Source: three-view drawing plus pictorial views. Frame: mm from the lowest corner of the part. A direction names the side the tool comes from. Give positions to 0.01 mm unless a question says otherwise; leave off trailing zeros. Order: outer loops, then holes, each group sorted by start corner. A loop starts at its lowest first (then second) coordinate and runs counter-clockwise, first axis right, second up. Notation, with made-up numbers: M -22.75,8 L 1.25,8 A29 ccw 1.25,37 Z; hole C 58,-39 d9. An arc over 180 degrees is marked long. Use CSV: the item, a comma, the result in double quotes. Start each with the question number.
Item 1: Section query A-A on y = 23. Return loops of the section in (x, z).
Item 2: Access query for the marked faces 1 and 2. Directions: +Z, -Z, +X, -X, +Y, -Y. A direction counts if a zero-diameter tool reaches every point of the face in a straight line with its end or side. Return the directions, or none.
Item 3: Section query B-B on z = 3.1. Return loops of the section in (x, y).
Item 4: Ray query, probe 1 along Y at (x, z) = (10, 2.35); probe 2 along Y at (x, z) = (14.75, 2.2); probe 3 along Y at (x, z) = (13, 4). Return the intervals inside material, ascending. Write a range as from..to.
Item 5: Section query C-C on x = 13.15. Return loops of the section in (y, z).
Item 6: Pull-direction query (X, two-part tool) for the marked faces 3, 4 and 5; classes: +X half, -X half, draft (parallel to the pull), parting line (faces both ways), or undercut.
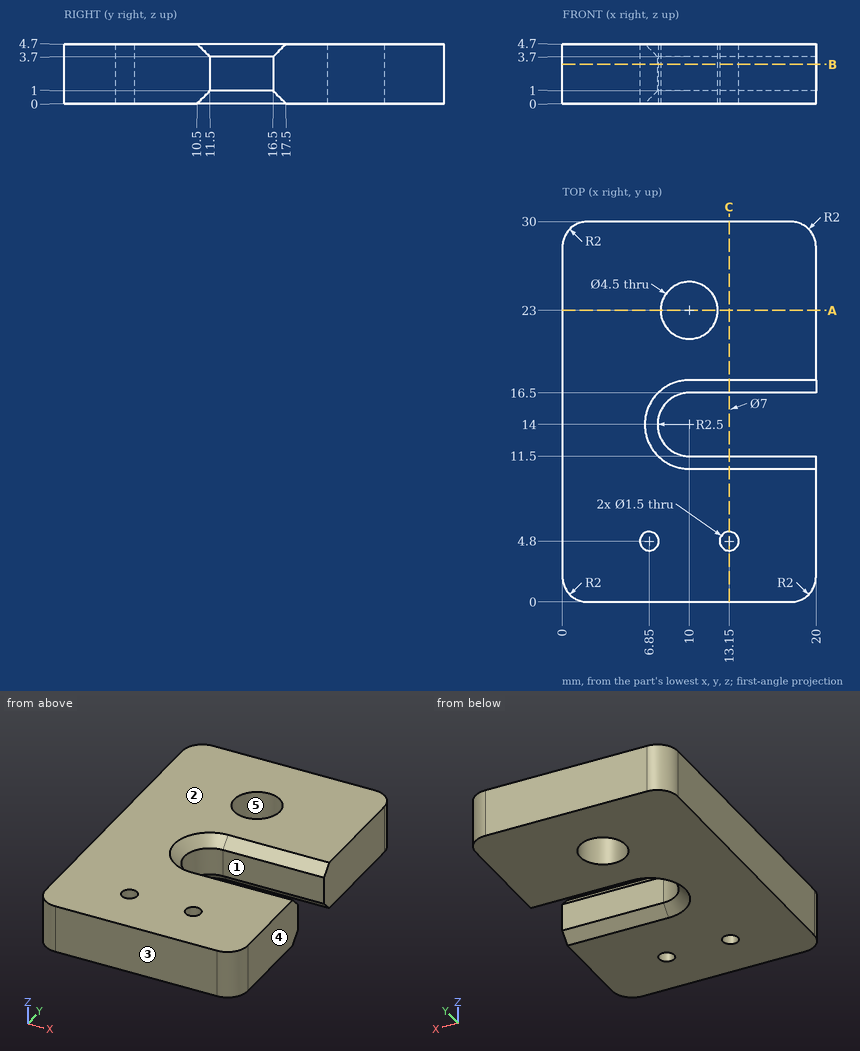
Verdict:
1,outline,"M 0,0 L 7.75,0 L 7.75,4.7 L 0,4.7 Z; M 12.25,0 L 20,0 L 20,4.7 L 12.25,4.7 Z"
2,face 1,"+Z, -Z, +X"
2,face 2,"+Z, +X, -X, +Y, -Y"
3,outline,"M 0,2 A2 ccw 2,0 L 18,0 A2 ccw 20,2 L 20,11.5 L 10,11.5 A2.5 cw 10,16.5 L 20,16.5 L 20,28 A2 ccw 18,30 L 2,30 A2 ccw 0,28 Z; hole C 6.85,4.8 d1.5; hole C 10,23 d4.5; hole C 13.15,4.8 d1.5"
4,probe 1,"0..11.5, 16.5..20.75, 25.25..30"
4,probe 2,"0..11.5, 16.5..30"
4,probe 3,"0..4.07, 5.53..11.2, 16.8..30"
5,outline,"M 0,0 L 4.05,0 L 4.05,4.7 L 0,4.7 Z; M 5.55,0 L 10.5,0 L 11.5,1 L 11.5,3.7 L 10.5,4.7 L 5.55,4.7 Z; M 16.5,1 L 17.5,0 L 30,0 L 30,4.7 L 17.5,4.7 L 16.5,3.7 Z"
6,face 3,"draft"
6,face 4,"+X half"
6,face 5,"undercut"
